```python
from build123d import *

# Parameters (mm, degrees)
P_IDAT_VYSUNUT_M1_DEPTH = 1


with BuildPart() as part:
    # Skica1 → Přidat vysunutím1 (new body)
    with BuildSketch(Plane.XY):
        with BuildLine():
            Line((-18, 24.202745422), (-30, 28.799160271))
            Line((-30, 28.799160271), (-30, 0))
            Line((-30, 0), (70, 0))
            Line((70, 0), (70, 57.421257865))
            Line((70, 57.421257865), (60.893124688, 57.421257865))
            Line((60.893124688, 57.421257865), (50, 42.815530581))
            add(Edge.make_bspline(
                [(-18, 24.202745422), (-15.420987086, 23.214894317), (-9.439226577, 21.709441745), (-0.04984208, 20.304879655), (10.115235915, 20.781402631), (20.26700575, 22.994551549), (34.677773963, 28.876632867), (44.35056656, 36.49037351), (50, 42.815530581)],
                knots=[0, 0, 0, 0, 0.110930708, 0.245725485, 0.379434234, 0.516153574, 0.660347153, 1, 1, 1, 1], degree=3))
        make_face()
    extrude(amount=P_IDAT_VYSUNUT_M1_DEPTH)


solid = part.part
```
Geometry check sheet. Reference: the model listing, model coordinates, mm. Give positions to 0.01 mm unless a question says otherwise; leave off trailing zeros. Order: outer loops, then holes, each group sorted by start corner. A loop starts at its lowest first (then second) coordinate and runs counter-clockwise, first axis right, second up. Notation, with made-up numbers: (5, 36.25) - (50, 36.25) arc R15 ccw to (50, 51.25) - close; hole circle Ø5 at (-2.5, -15.5). An arc over 180 degrees is marked (long way). Answer in a Markdown table with one row per item. Add a question column.
Q1. Cross-section at A-A, the plane y = 48. Enter the section's corners in (x, z), then the cut area to 3 significant figures.
Q2. Material ranges on probe 1 along X at (y, z) = (41.5, 0.95); probe 2 along Y at (x, z) = (56.5, 0.65); probe 3 along X at (y, z) = (45, 0.6), recorded low to high. Write a range as from..to.
Q3. Mould release check, pull along X, two halves, no side actions. Record for faces 1 (the flat face through (-23.92, 26.47, 0.49)), 2 (the flat face through (55.52, 50.22, 0.49)), 3 (the flat face through (30, 16, 0)): pulls with the +X half, pulls with the -X half, needs draft (parallel to the pull), parting line crosses it, or undercut.
Check values:
| question | item | result |
|---|---|---|
| 1 | outline | (53.87, 0) - (70, 0) - (70, 1) - (53.87, 1) - close |
| 1 | area | 16.1 mm^2 |
| 2 | probe 1 | x = 48.8..70 |
| 2 | probe 2 | y = 0..51.53 |
| 2 | probe 3 | x = 51.63..70 |
| 3 | face 1 | undercut |
| 3 | face 2 | pulls with the -X half |
| 3 | face 3 | needs draft |
